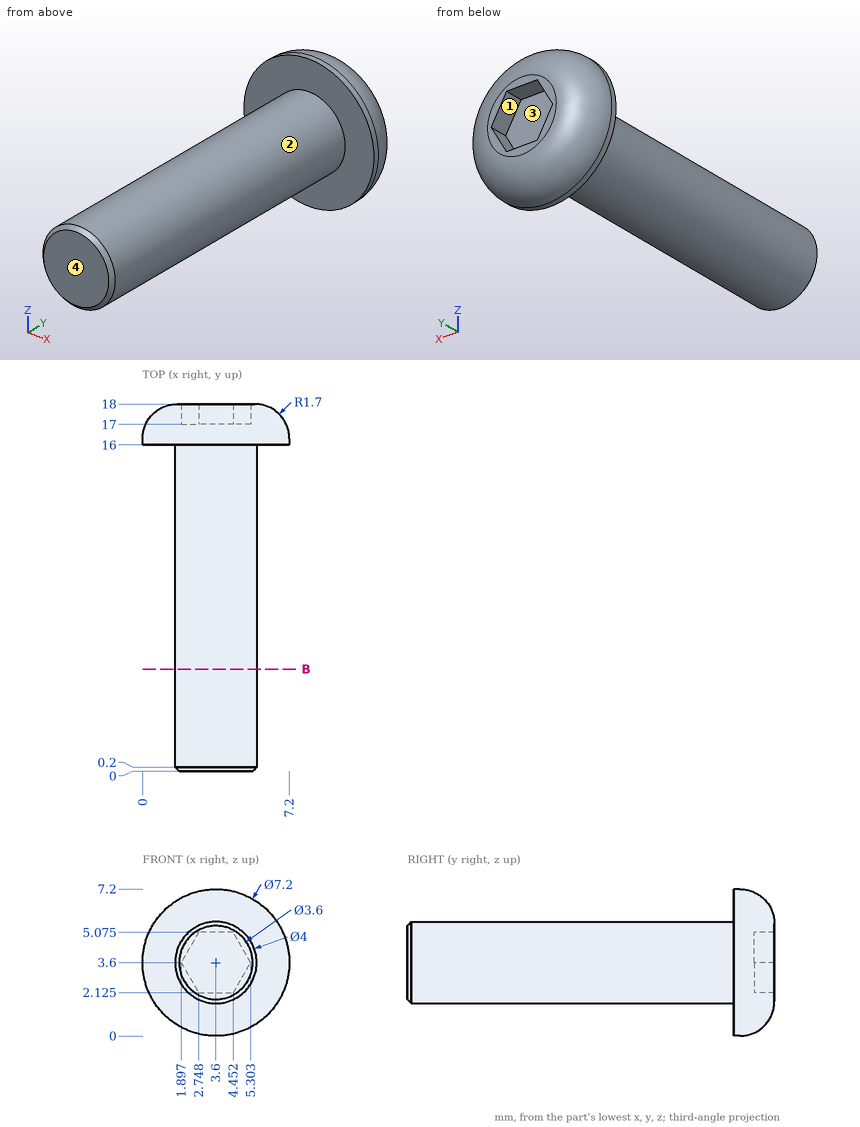
Geometry check sheet. Reference: drawing and pictorial views, mm from the part's lowest x, y, z. Round coordinates to 2 decimals unless told otherwise and drop trailing zeros. Loops run counter-clockwise (first coordinate to the right, second up) from the corner with the lowest first, then second, coordinate; pieces in that order, holes last. Notation, with made-up numbers: M 27.25,-20 L 74.25,-20 A32 ccw 74.25,6 Z; hole C 43,16.5 d1. An arc over 180 degrees is marked long. Return JSON: item names as keys, results as strings. Group by question number.
(1) Mould release check, pull along X, two halves, no side actions. Record for the marked faces 1, 2, 3 and 4: pulls with the +X half, pulls with the -X half, needs draft (parallel to the pull), parting line crosses it, or undercut.
(2) Scan lines: line 1 along Z through (x, y) = (2.25, 13.25) (1 decimal); line 2 along X through (y, z) = (12, 3.5); line 3 along Y through (x, z) = (2.75, 3.25). Record each from-to range of solid material in increasing order. Write a range as [from, to].
(3) Go/stop test with flat-tipped pins: pin 1 (1.5 mm diameter, centred on y = 13, z = 5.5, fed in from -X); pin 2 (4 mm diameter, centred on x = 1, z = 5, fed in from -Y); pin 3 (0.8 mm diameter, centred on x = 3.5, y = 17.5, fed in from +Z); pin 4 (0.9 mm diameter, centred on x = 4.5, z = 3.5, fed in from +Y). Record where each tip stops, or that it passes through.
(4) Section check B-B, the plane y = 5. Enter the section's corners in (x, z).
Data:
{
 "1": {"face 1": "undercut", "face 2": "parting line crosses it", "face 3": "undercut", "face 4": "needs draft"},
 "2": {"line 1": "[2.1, 5.1]", "line 2": "[1.6, 5.6]", "line 3": "[0, 17]"},
 "3": {"pin 1": "x = 1.96", "pin 2": "y = 0", "pin 3": "z = 7", "pin 4": "y = 17"},
 "4": {"outline": "C 3.6,3.6 d4"}
}
